```python
from build123d import *

# Parameters (mm, degrees)
SKETCH1_R           = 2.5
BOSS_EXTRUDE1_DEPTH = 250


with BuildPart() as part:
    # Sketch1 → Boss-Extrude1 (new body)
    with BuildSketch(Plane.XY):
        with BuildLine():
            Line((-4.725542729, -10), (-3.125, -8.2))
            Line((-3.125, -8.2), (-5.5, -8.2))
            Line((-5.5, -8.2), (-5.5, -6.560660172))
            Line((-5.5, -6.560660172), (-2.539339828, -3.6))
            Line((-2.539339828, -3.6), (2.539339828, -3.6))
            Line((2.539339828, -3.6), (5.5, -6.560660172))
            Line((5.5, -6.560660172), (5.5, -8.2))
            Line((5.5, -8.2), (3.125, -8.2))
            Line((3.125, -8.2), (4.434457271, -10))
            Line((4.434457271, -10), (8, -10))
            ThreePointArc((8, -10), (9.414213562, -9.414213562), (10, -8))
            Line((10, -8), (10, -4.434457271))
            Line((10, -4.434457271), (8.2, -3.125))
            Line((8.2, -3.125), (8.2, -5.5))
            Line((8.2, -5.5), (6.560660172, -5.5))
            Line((6.560660172, -5.5), (3.6, -2.539339828))
            Line((3.6, -2.539339828), (3.6, 2.539339828))
            Line((3.6, 2.539339828), (6.560660172, 5.5))
            Line((6.560660172, 5.5), (8.2, 5.5))
            Line((8.2, 5.5), (8.2, 3.125))
            Line((8.2, 3.125), (10, 4.725542729))
            Line((10, 4.725542729), (10, 8))
            ThreePointArc((10, 8), (9.414213562, 9.414213562), (8, 10))
            Line((8, 10), (4.725542729, 10))
            Line((4.725542729, 10), (3.125, 8.2))
            Line((3.125, 8.2), (5.5, 8.2))
            Line((5.5, 8.2), (5.5, 6.560660172))
            Line((5.5, 6.560660172), (2.539339828, 3.6))
            Line((2.539339828, 3.6), (-2.539339828, 3.6))
            Line((-2.539339828, 3.6), (-5.5, 6.560660172))
            Line((-5.5, 6.560660172), (-5.5, 8.2))
            Line((-5.5, 8.2), (-3.125, 8.2))
            Line((-3.125, 8.2), (-4.434457271, 10))
            Line((-4.434457271, 10), (-8, 10))
            ThreePointArc((-8, 10), (-9.414213562, 9.414213562), (-10, 8))
            Line((-10, 8), (-10, 4.434457271))
            Line((-10, 4.434457271), (-8.2, 3.125))
            Line((-8.2, 3.125), (-8.2, 5.5))
            Line((-8.2, 5.5), (-6.560660172, 5.5))
            Line((-6.560660172, 5.5), (-3.6, 2.539339828))
            Line((-3.6, 2.539339828), (-3.6, -2.539339828))
            Line((-3.6, -2.539339828), (-6.560660172, -5.5))
            Line((-6.560660172, -5.5), (-8.2, -5.5))
            Line((-8.2, -5.5), (-8.2, -3.125))
            Line((-8.2, -3.125), (-10, -4.725542729))
            Line((-10, -4.725542729), (-10, -8))
            ThreePointArc((-10, -8), (-9.414213562, -9.414213562), (-8, -10))
            Line((-8, -10), (-4.725542729, -10))
        make_face()
        Circle(SKETCH1_R, mode=Mode.SUBTRACT)
    extrude(amount=BOSS_EXTRUDE1_DEPTH)


solid = part.part
```
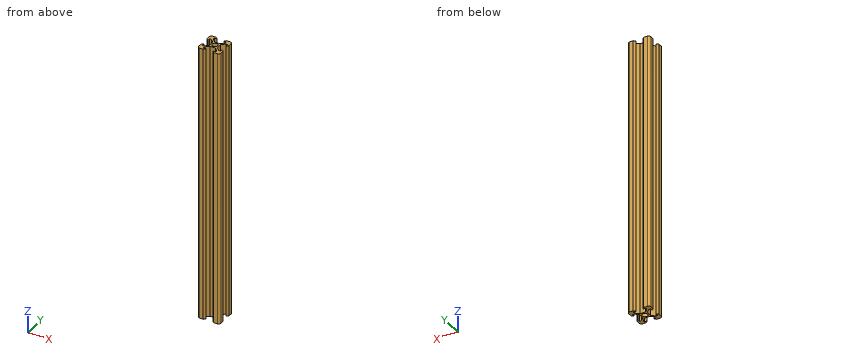
Geometry: final body of the model. Coordinates: model frame, mm. Coordinates: 2 decimals unless noted, no trailing zeros. Order: outer loops, then holes, each group sorted by start corner. A loop starts at its lowest first (then second) coordinate and runs counter-clockwise, first axis right, second up.
Item 1: Section query A-A (y = 0). Output: boundary loops of the cut face in (x, z), then the cut area to 3 significant figures.
Answer:
outline: (-3.6, 0) - (-2.5, 0) - (-2.5, 250) - (-3.6, 250) - close; (2.5, 0) - (3.6, 0) - (3.6, 250) - (2.5, 250) - close
area: 550 mm2
Item 2: Material intervals for line 1 along Y through (x, z) = (0, 81.5); line 2 along Y through (x, z) = (-8, 128); line 3 along X through (y, z) = (-5.25, 64), sorted ascending.
Answer:
line 1: y = -3.6 to -2.5, 2.5 to 3.6
line 2: y = -10 to -5.5, 5.5 to 10
line 3: x = -10 to -8.2, -6.31 to -4.19, 4.19 to 6.31, 8.2 to 10
Item 3: Contact query for flat-ended pins moving along their axis: P1, Ø1, axis at x = 1, z = 51.5, coming from the +Y side; P2, Ø1, axis at x = 1, z = 99.5, coming from the -Y side; P3, Ø1.2, axis at y = 4, z = 123, coming from the +X side; P4, Ø1, axis at x = -2.5, y = 7.5, coming from the -Z side. Output: stop coordinate, or through.
Answer:
P1: stops at y = 3.6
P2: stops at y = -3.6
P3: stops at x = 9.86
P4: passes through
